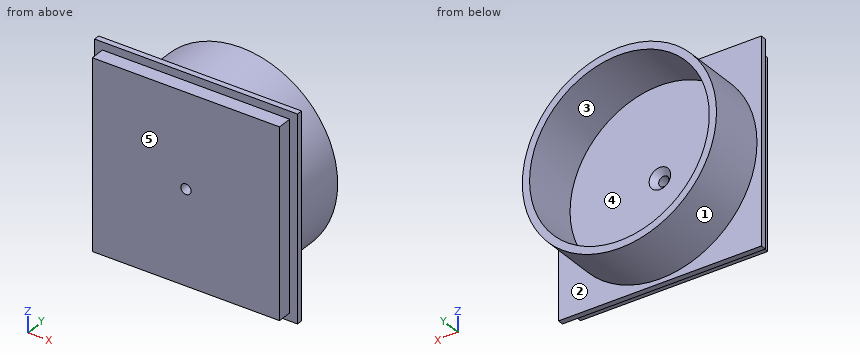
from build123d import *

# Parameters (mm, degrees)
SKETCH1_W                                       = 82.042
SKETCH1_H                                       = 82.042
BOSS_EXTRUDE1_DEPTH                             = 6.35
SKETCH3_W                                       = 88.9
SKETCH3_H                                       = 88.9
BOSS_EXTRUDE3_DEPTH                             = 2.54
SKETCH4_R                                       = 2.25
CUT_EXTRUDE1_DEPTH                              = 9.89
SKETCH5_R                                       = 42.545
SKETCH5_R_2                                     = 39.37
BOSS_EXTRUDE4_DEPTH                             = 25.4
CSK_FOR_M4_FLAT_HEAD_MACHINE_SCREW1_D           = 4.5
CSK_FOR_M4_FLAT_HEAD_MACHINE_SCREW1_DEPTH       = 3.99999
CSK_FOR_M4_FLAT_HEAD_MACHINE_SCREW1_CSINK_D     = 9.4
CSK_FOR_M4_FLAT_HEAD_MACHINE_SCREW1_CSINK_ANGLE = 90
CSK_FOR_M4_FLAT_HEAD_MACHINE_SCREW1_TIP         = 1.351936393


with BuildPart() as part:
    # Sketch1 → Boss-Extrude1 (new body)
    with BuildSketch(Plane(origin=(0, 0, 0), x_dir=(1, 0, 0), z_dir=(0, 1, 0))):
        with Locations((41.021, 41.021)):
            Rectangle(SKETCH1_W, SKETCH1_H)
    extrude(amount=BOSS_EXTRUDE1_DEPTH)

    # Sketch3 → Boss-Extrude3 (add)
    with BuildSketch(Plane(origin=(0, 6.35, 0), x_dir=(1, 0, 0), z_dir=(0, 1, 0))):
        with Locations((41.021, 41.021)):
            Rectangle(SKETCH3_W, SKETCH3_H)
    extrude(amount=BOSS_EXTRUDE3_DEPTH)

    # Sketch4 → Cut-Extrude1 (cut, through all)
    with BuildSketch(Plane(origin=(0, 8.89, 0), x_dir=(1, 0, 0), z_dir=(0, 1, 0))):
        with Locations((41.021, 41.021)):
            Circle(SKETCH4_R)
    extrude(amount=-CUT_EXTRUDE1_DEPTH, mode=Mode.SUBTRACT)

    # Sketch5 → Boss-Extrude4 (add)
    with BuildSketch(Plane(origin=(0, 8.89, 0), x_dir=(1, 0, 0), z_dir=(0, 1, 0))):
        with Locations((41.021, 41.021)):
            Circle(SKETCH5_R)
        with Locations((41.021, 41.021)):
            Circle(SKETCH5_R_2, mode=Mode.SUBTRACT)
    extrude(amount=BOSS_EXTRUDE4_DEPTH)

    # CSK for M4 Flat Head Machine Screw1
    with Locations(Plane(origin=(0, 8.89, 0), x_dir=(1, 0, 0), z_dir=(0, 1, 0))):
        with Locations((41.021, 41.021)):
            CounterSinkHole(CSK_FOR_M4_FLAT_HEAD_MACHINE_SCREW1_D / 2, CSK_FOR_M4_FLAT_HEAD_MACHINE_SCREW1_CSINK_D / 2, depth=CSK_FOR_M4_FLAT_HEAD_MACHINE_SCREW1_DEPTH, counter_sink_angle=CSK_FOR_M4_FLAT_HEAD_MACHINE_SCREW1_CSINK_ANGLE)
            with Locations((0, 0, -(CSK_FOR_M4_FLAT_HEAD_MACHINE_SCREW1_DEPTH + CSK_FOR_M4_FLAT_HEAD_MACHINE_SCREW1_TIP / 2))):  # 118° drill point
                Cone(0, CSK_FOR_M4_FLAT_HEAD_MACHINE_SCREW1_D / 2, CSK_FOR_M4_FLAT_HEAD_MACHINE_SCREW1_TIP, mode=Mode.SUBTRACT)


solid = part.part
Build history of the part. All positions in model axes, mm. Face numbers are marked on the shaded views. A direction names the side the tool comes from. Round coordinates to 2 decimals unless told otherwise and drop trailing zeros. Loops run counter-clockwise (first coordinate to the right, second up) from the corner with the lowest first, then second, coordinate; pieces in that order, holes last. Notation, with made-up numbers: (-31, -11.5) -> (-23, -11.5) arc R25 cw to (-23, 11.5) -> close; hole circle Ø1 at (24.5, -21). An arc over 180 degrees is marked (long way). Use CSV: the item, a comma, the result in double quotes. Start each with the question number.
Q1. Which spindle directions (+Z, -Z, +X, -X, +Y, -Y) get a long thin tool onto all of the face, cutting with end or side? Do the marked faces 4 and 5. Say none if no direction does.
Q2. Drill centre lines: L1, parallel to Z at x = 15, y = 1; L2, parallel to Y at x = 30, z = -47.5; L3, parallel to Z at x = 41, y = 25. Where is each one in solid material? Low to high.
Q3. Saw through at A-A on x = 10. Give the cut face in (y, z), and give its area (3 significant figures).
Q4. Flat gauge pins, fed straight in: pin 1 Ø7 at (x, y) = (57, 2) entering from -Z; pin 2 Ø10 at (x, z) = (32, -19.5) entering from +Y; pin 3 Ø5 at (x, y) = (30.5, 2.5) entering from +Z. Where does each tip first touch, or does it go through?
Q5. Saw through at D-D on y = 28.5. Give the cut face in (x, z) (3 decimals).
Q6. Saw through at C-C on y = 2. Give the cut face in (x, z), and give its area (4 significant figures).
Q7. Mould opens along X. For the marked faces 1, 2 and 3 say: +X half, -X half, draft (parallel to the pull), parting line (faces both ways), or undercut.
Q8. Saw through at B-B on z = -71. Give the cut face in (x, y).
Solutions:
1,face 4,"+Y"
1,face 5,"+Z, -Z, +X, -X, -Y"
2,L1,"z = -82.04 to 0"
2,L2,"y = 0 to 8.89"
2,L3,"z = -83.57 to -80.39, -1.65 to 1.52"
3,outline,"(0, -82.04) -> (6.35, -82.04) -> (6.35, -85.47) -> (8.89, -85.47) -> (8.89, -70.14) -> (34.29, -70.14) -> (34.29, -65.26) -> (8.89, -65.26) -> (8.89, -16.78) -> (34.29, -16.78) -> (34.29, -11.9) -> (8.89, -11.9) -> (8.89, 3.43) -> (6.35, 3.43) -> (6.35, 0) -> (0, 0) -> close"
3,area,"994 mm^2"
4,pin 1,"stops at z = -82.04"
4,pin 2,"stops at y = 8.89"
4,pin 3,"stops at z = 0"
5,outline,"circle Ø85.09 at (41.021, -41.021); hole circle Ø78.74 at (41.021, -41.021)"
6,outline,"(0, -82.04) -> (82.04, -82.04) -> (82.04, 0) -> (0, 0) -> close; hole circle Ø4.5 at (41.02, -41.02)"
6,area,"6,715 mm^2"
7,face 1,"parting line"
7,face 2,"draft"
7,face 3,"undercut"
8,outline,"(-3.43, 6.35) -> (0, 6.35) -> (0, 0) -> (82.04, 0) -> (82.04, 6.35) -> (85.47, 6.35) -> (85.47, 8.89) -> (71.21, 8.89) -> (71.21, 34.29) -> (66.54, 34.29) -> (66.54, 8.89) -> (15.5, 8.89) -> (15.5, 34.29) -> (10.83, 34.29) -> (10.83, 8.89) -> (-3.43, 8.89) -> close"
